Source: CAD feature listing. Evaluate the final solid. Frame: model axes, mm. A direction names the side the tool comes from. Coordinates: 2 decimals unless noted, no trailing zeros. Write each loop counter-clockwise with the first axis right and the second up, starting at its lowest first coordinate (ties: lowest second). Pieces come first, ordered by that corner, then holes. Notation, with made-up numbers: (-26.5, 8.25) - (0.5, 8.25) arc R23 ccw to (0.5, 40.25) - close; hole circle Ø2 at (-3.75, 87). An arc over 180 degrees is marked (long way). One line per item, written item: value.
Autodesk Inventor part; units mm, degrees
ref_plane "YZ Plane" through (0, 0, 0) normal (1, 0, 0) x (0, 1, 0)
ref_plane "XZ Plane" through (0, 0, 0) normal (0, 1, 0) x (-1, 0, 0)
ref_plane "XY Plane" through (0, 0, 0) normal (0, 0, 1) x (1, 0, 0)
sketch "Sketch1" plane through (0, 0, 0) normal (0, 0, 1) x (1, 0, 0)
  line L0 (7.5, 7.5) -> (-7.5, 7.5)
  line L1 (7.5, 7.5) -> (-7.5, 7.5)
  line L2 (-7.5, 7.5) -> (-7.5, -7.5)
  line L3 (-7.5, -7.5) -> (7.5, -7.5)
  line L4 (7.5, -7.5) -> (7.5, 7.5)
  line L5 (-8.5, 8.5) -> (8.5, 8.5)
  line L6 (8.5, 8.5) -> (8.5, -8.5)
  line L7 (8.5, -8.5) -> (-8.5, -8.5)
  line L8 (-8.5, -8.5) -> (-8.5, 8.5)
  point P0 (0, 0)
extrude "Extrusion1" add sketch "Sketch1" along normal blind 1 contours L4 L3 L2 L0 | L5 L6 L7 L8
sketch "Sketch2" plane through (0, 0, 0) normal (0, 0, -1) x (-1, 0, 0)
  line L0 (-7.5, 7.5) -> (7.5, 7.5)
  line L1 (7.5, 7.5) -> (7.5, -7.5)
  line L2 (7.5, -7.5) -> (-7.5, -7.5)
  line L3 (-7.5, -7.5) -> (-7.5, 7.5)
  line L4 (8.5, 8.5) -> (-8.5, 8.5)
  line L5 (-8.5, 8.5) -> (-8.5, -8.5)
  line L6 (-8.5, -8.5) -> (8.5, -8.5)
  line L7 (8.5, -8.5) -> (8.5, 8.5)
  line L8 (-7.5, -7.5) -> (-5.5, -7.5)
  line L9 (-5.5, -7.5) -> (-5.5, 7.5)
  line L10 (-5.5, 7.5) -> (-7.5, 7.5)
  line L11 (-7.5, 7.5) -> (-7.5, -7.5)
  line L12 (7.5, 7.5) -> (5.5, 7.5)
  line L13 (5.5, 7.5) -> (5.5, -7.5)
  line L14 (5.5, -7.5) -> (7.5, -7.5)
  line L15 (7.5, -7.5) -> (7.5, 7.5)
  point P0 (0, 0)
  dimension "d2" = 2
  dimension "d3" = 2
extrude "Extrusion2" add sketch "Sketch2" along normal blind 4 contours L0 L9 L2 L3 | L0 L1 L2 L13
thicken "Thicken1" operation add thickness 0.1 both sides no extend neighbours yes toward (0, -1, 0) faces at (6.1667, 7.5, -1.3333) (7.5, 2.5, -1.3333) (6.8333, -7.5, -1.3333)
thicken "Thicken2" operation add thickness 0.1 both sides no extend neighbours yes toward (0, 1, 0) faces at (-6.1667, -7.5, -1.3333) (-7.5, -2.5, -1.3333) (-6.8333, 7.5, -1.3333)
properties part number "hull_cover_cover"
1) Contact query for flat-ended pins moving along their axis: P1, Ø1, axis at x = -6.5, z = -1, coming from the -Y side; P2, Ø1.2, axis at y = 1, z = -1.5, coming from the -X side; P3, Ø1.2, axis at y = -3.5, z = -1, coming from the +X side. Output: stop coordinate, or through.
Values found:
P1: y = -7.4
P2: x = -7.4
P3: x = 7.4
2) Reachability of faces 4 (the flat face through (5.5, 0, -2)), 5 (the flat face through (-7.4, 0, -2)), 6 (the flat face through (6, -7.4, -2)), 7 (the flat face through (7.4, 0, -2)), 8 (the flat face through (6, 7.4, -2)) from +Z, -Z, +X, -X, +Y, -Y: full face, straight path, thin tool, end or side. Return the list, or none.
Values found:
face 4: -Z, +Y, -Y
face 5: -Z, -X, +Y, -Y
face 6: -Z, +X, -X, -Y
face 7: -Z, +X, +Y, -Y
face 8: -Z, +X, -X, +Y
3) Section query C-C on y = -4. Output: boundary loops of the cut face in (x, z), then the cut area to 3 significant figures.
Values found:
outline: (-8.5, 0) - (-7.4, 0) - (-7.4, -4) - (-5.5, -4) - (-5.5, 0) - (5.5, 0) - (5.5, -4) - (7.4, -4) - (7.4, 0) - (8.5, 0) - (8.5, 1) - (-8.5, 1) - close
area: 32.2 mm2
4) Material intervals for line 1 (X direction, y = 3.75, z = -2); line 2 (Z direction, x = 0.25, y = 3.25); line 3 (Y direction, x = 7.25, z = -2.6), sorted ascending.
Values found:
line 1: -7.4 to -5.5, 5.5 to 7.4
line 2: 0 to 1
line 3: -7.4 to 7.4
5) Draft query along X for faces 1 (the flat face through (0, 0, 0)), 2 (the flat face through (-8.5, -0.1, 0.5)), 3 (the flat face through (-6, 7.4, -2)). Return one class per face: released by +X, released by -X, zero draft, split by the parting line, or undercut.
Values found:
face 1: undercut
face 2: released by -X
face 3: zero draft
6) Section query B-B on x = -6.75. Output: boundary loops of the cut face in (y, z), then the cut area to 3 significant figures.
Values found:
outline: (-8.5, 0) - (-7.4, 0) - (-7.4, -4) - (7.4, -4) - (7.4, 0) - (8.5, 0) - (8.5, 1) - (-8.5, 1) - close
area: 76.2 mm2
7) Section query D-D on x = -2. Output: boundary loops of the cut face in (y, z), then the cut area to 3 significant figures.
Values found:
outline: (-8.5, 0) - (8.5, 0) - (8.5, 1) - (-8.5, 1) - close
area: 17.0 mm2
8) Section query A-A on z = -0.95. Output: boundary loops of the cut face in (x, y).
Values found:
outline: (-7.4, -7.4) - (-5.5, -7.4) - (-5.5, 7.4) - (-7.4, 7.4) - close; (5.5, -7.4) - (7.4, -7.4) - (7.4, 7.4) - (5.5, 7.4) - close
